```python
from build123d import *

# Parameters (mm, degrees)
EXTRUDE_1_DEPTH     = 6
SKETCH_5_R          = 3.5
CUT_EXTRUDE_2_DEPTH = 7
CHAMFER_1_SIZE      = 0.5


with BuildPart() as part:
    # Эскиз1 → Вытянуть1 (new body)
    with BuildSketch(Plane.XY):
        Polygon((-3.019213701, 6.315405658), (-6.978908586, 0.542987065), (-3.959694885, -5.772418593), (3.019213701, -6.315405658), (6.978908586, -0.542987065), (3.959694885, 5.772418593), align=None)
    extrude(amount=EXTRUDE_1_DEPTH)

    # Вырез-По траектории1: sweep along a path in Эскиз3
    with BuildLine(Plane(origin=(0, 0, 0), x_dir=(-1, 0, 0), z_dir=(0, 0, -1))) as sweep_1_path:
        CenterArc((0, 0), 4.80754516, 0, 360)
    # Эскиз4 → Вырез-По траектории1 (sweep, cut)
    with BuildSketch(Plane(origin=(0, 0, 0), x_dir=(1, 0, 0), z_dir=(0, 1, 0))):
        Polygon((-5.152045548, 0), (-8.017144415, -0.472678529), (-8.017144415, 0.689853389), align=None)
    sweep_1 = sweep(path=sweep_1_path.line, mode=Mode.SUBTRACT)

    # Зеркальное отражение1: Вырез-По траектории1 across plane
    add(sweep_1.mirror(Plane(origin=(0, 0, 3), x_dir=(1, 0, 0), z_dir=(0, 0, -1))), mode=Mode.SUBTRACT)

    # Эскиз5 → Вытянуть2 (cut, through all)
    with BuildSketch(Plane.XY.offset(6)):
        Circle(SKETCH_5_R)
    extrude(amount=-CUT_EXTRUDE_2_DEPTH, mode=Mode.SUBTRACT)

    # Фаска1
    chamfer_1_edges = [part.edges().sort_by_distance(p)[0] for p in [
        (-3.5, 0, 0),
    ]]
    chamfer(chamfer_1_edges, length=CHAMFER_1_SIZE)


solid = part.part
```
Part model, mm, in its own coordinate system. Give positions to 0.01 mm unless a question says otherwise; leave off trailing zeros. Order: outer loops, then holes, each group sorted by start corner. A loop starts at its lowest first (then second) coordinate and runs counter-clockwise, first axis right, second up. Notation, with made-up numbers: M 63,-34.5 L 110,-34.5 A11 ccw 110,-17.5 Z; hole C -35,23.5 d3. An arc over 180 degrees is marked long. Use a Markdown table: item, result. Add a question column.
(1) Saw through at C-C, the plane z = 1.6. Give the cut face in (x, y).
(2) Mould opens along Y. For faces 1 (the face through (4.97, -3.47, 2.96)), 2 (the face through (0, 4, 6)), 3 (the face through (3.233, -1.341, 3.288)) say: +Y half, -Y half, draft (parallel to the pull), parting line (faces both ways), or undercut.
(3) Probe line 1 along X through (y, z) = (2.75, 4); line 2 along X through (y, z) = (-1.5, 2.8); line 3 along Y through (x, z) = (-0.5, 5.05). List the from-to ranges inside material, lowest first. Write a range as [from, to].
(4) Saw through at B-B, the plane y = 0. Give the cut face in (x, z), and give its area (3 significant figures).
(5) Saw through at A-A, the plane x = 0. Give the cut face in (y, z).
(6) Drop flat-ended pins along their axis: P1, Ø1, axis at x = 5.5, y = 1.5, coming from the -Z side; P2, Ø1, axis at x = -0.5, z = 4, coming from the -Y side; P3, Ø1.5, axis at y = 2.5, z = 2.5, coming from the -X side. Give the stop position or say it passes through.
Answer key:
| question | item | result |
|---|---|---|
| 1 | outline | M -6.98,0.54 L -3.96,-5.77 L 3.02,-6.32 L 6.98,-0.54 L 3.96,5.77 L -3.02,6.32 Z; hole C 0,0 d7 |
| 2 | face 1 | -Y half |
| 2 | face 2 | draft |
| 2 | face 3 | undercut |
| 3 | line 1 | [-5.46, -2.17], [2.17, 5.4] |
| 3 | line 2 | [-6, -3.16], [3.16, 6.32] |
| 3 | line 3 | [-6.04, -3.46], [3.46, 6.12] |
| 4 | outline | M -6.72,0.26 L -5.15,0 L -4,0 L -3.5,0.5 L -3.5,6 L -5.15,6 L -6.72,5.74 Z; M 3.5,0.5 L 4,0 L 5.15,0 L 6.72,0.26 L 6.72,5.74 L 5.15,6 L 3.5,6 Z |
| 4 | area | 37.6 mm^2 |
| 5 | outline | M -6.08,0.15 L -5.15,0 L -4,0 L -3.5,0.5 L -3.5,6 L -5.15,6 L -6.08,5.85 Z; M 3.5,0.5 L 4,0 L 5.15,0 L 6.08,0.15 L 6.08,5.85 L 5.15,6 L 3.5,6 Z |
| 6 | P1 | z = 0.01 |
| 6 | P2 | y = -6.08 |
| 6 | P3 | x = -6.15 |
